Design review of the part built by this model. Coordinates are the model's own, in mm. A direction names the side the tool comes from. Coordinates: 2 decimals unless noted, no trailing zeros. Loops run counter-clockwise (first coordinate to the right, second up) from the corner with the lowest first, then second, coordinate; pieces in that order, holes last. Notation, with made-up numbers: (-39.75, 64.25) - (-2.75, 64.25) arc R20 ccw to (-2.75, 87.25) - close; hole circle Ø5 at (69.5, 29.25). An arc over 180 degrees is marked (long way). Use one line per item in the form item = value. Start each with the question number.
(1) Add section A-A (x = -1). State the section outline as (y, z) points, plus the area to 3 significant figures.
(2) For L1, parallel to X at y = 1.7, z = -4; L2, parallel to X at y = 3.75, z = -0.75; L3, parallel to Z at x = -0.5, y = 1.5, list the stretches that pass through material, from the lowest coordinate up.
(3) Tool access review of faces 1 (the face through (-4.5, 2, 0)), 2 (the face through (3.5, 2, 2)): name each direction out of +Z, -Z, +X, -X, +Y, -Y from which nothing blocks a thin tool from reaching the whole face with its end or side.
(4) Add section C-C (y = 0.6). State the section outline as (x, z) points.
(5) Add section D-D (z = -4). State the section outline as (x, y) points, plus the area to 3 significant figures.
(6) Add section B-B (x = 0). State the section outline as (y, z) points.
(7) Clearance check with a flat-ended pin moving along its axis: pin 1 Ø1 at (x, z) = (-0.5, -3.5) entering from -Y. State where the tip first meets the part, or that it passes through.
(8) The part is to be moulded in two halves that separate along Z. For faces 3 (the face through (0, 2, -2)), 4 (the face through (4.5, 2, 0)), 5 (the face through (4.199, 2.415, 5.715)), 6 (the face through (-3.215, 2.348, -1.699)), say which applies: pulls with the +Z half, pulls with the -Z half, needs draft (parallel to the pull), parting line crosses it, or undercut.
```python
from build123d import *

# Parameters (mm, degrees)
SKETCH1_W                           = 9
SKETCH1_H                           = 12
EXTRUDE1_DEPTH                      = 4.7625
SKETCH2_W                           = 7
SKETCH2_H                           = 7
EXTRUDE2_DEPTH                      = 5.7625
F_0_80_TAPPED_HOLE1_D               = 1.19126
F_3_32_0_09375_DIAMETER_HOLE1_D     = 2.38125
F_3_32_0_09375_DIAMETER_HOLE1_DEPTH = 10
F_3_32_0_09375_DIAMETER_HOLE1_TIP   = 0.715399675
FILLET7_R                           = 1


with BuildPart() as part:
    # Sketch1 → Extrude1 (new body)
    with BuildSketch(Plane(origin=(0, 0, 0), x_dir=(1, 0, 0), z_dir=(0, 1, 0))):
        Rectangle(SKETCH1_W, SKETCH1_H)
    extrude(amount=EXTRUDE1_DEPTH)

    # Sketch2 → Extrude2 (cut, through all)
    with BuildSketch(Plane(origin=(0, 4.7625, 0), x_dir=(1, 0, 0), z_dir=(0, 1, 0))):
        with Locations((0, -1.5)):
            Rectangle(SKETCH2_W, SKETCH2_H)
    extrude(amount=-EXTRUDE2_DEPTH, mode=Mode.SUBTRACT)

    # #0-80 Tapped Hole1 (through all)
    with Locations(Plane(origin=(0, 4.7625, -4), x_dir=(0, 0, 1), z_dir=(0, 1, 0))):
        with Locations((0, 0)):
            Hole(F_0_80_TAPPED_HOLE1_D / 2)

    # 3/32 (0.09375) Diameter Hole1
    with Locations(Plane(origin=(-2.5, 4.7625, -4), x_dir=(0, 0, 1), z_dir=(0, 1, 0))):
        with Locations((0, 0), (0, 5)):
            Hole(F_3_32_0_09375_DIAMETER_HOLE1_D / 2, depth=F_3_32_0_09375_DIAMETER_HOLE1_DEPTH)
            with Locations((0, 0, -(F_3_32_0_09375_DIAMETER_HOLE1_DEPTH + F_3_32_0_09375_DIAMETER_HOLE1_TIP / 2))):  # 118° drill point
                Cone(0, F_3_32_0_09375_DIAMETER_HOLE1_D / 2, F_3_32_0_09375_DIAMETER_HOLE1_TIP, mode=Mode.SUBTRACT)

    # Fillet7
    fillet7_edges = [part.edges().sort_by_distance(p)[0] for p in [
        (-3.5, 2.38125, 5),
        (-3.5, 2.38125, -2),
        (3.5, 2.38125, -2),
        (3.5, 2.38125, 5),
        (-4.5, 2.38125, -6),
        (4.5, 2.38125, -6),
        (4.5, 2.38125, 6),
        (-4.5, 2.38125, 6),
    ]]
    fillet(fillet7_edges, radius=FILLET7_R)


solid = part.part
```
Computed values:
q1.outline = (0, -6) - (4.76, -6) - (4.76, -2) - (0, -2) - close; (0, 5) - (4.76, 5) - (4.76, 6) - (0, 6) - close
q1.area = 23.8 mm^2
q2.L1 = -4.5 to -3.69, -1.31 to -0.6, 0.6 to 1.31, 3.69 to 4.5
q2.L2 = -4.5 to -3.5, 3.5 to 4.5
q2.L3 = -6 to -4.32, -3.68 to -2, 5 to 6
q3.face_1 = +Z, -Z, -X, +Y, -Y
q3.face_2 = +Y, -Y
q4.outline = (-4.5, -5) arc R1 ccw to (-3.5, -6) - (3.5, -6) arc R1 ccw to (4.5, -5) - (4.5, 5) arc R1 ccw to (3.5, 6) - (-3.5, 6) arc R1 ccw to (-4.5, 5) - close; hole circle Ø2.38 at (-2.5, -4); hole (-3.5, -1) arc R1 ccw to (-2.5, -2) - (2.5, -2) arc R1 ccw to (3.5, -1) - (3.5, 4) arc R1 ccw to (2.5, 5) - (-2.5, 5) arc R1 ccw to (-3.5, 4) - close; hole circle Ø1.19 at (0, -4); hole circle Ø2.38 at (2.5, -4)
q5.outline = (-4.5, 0) - (-3.69, 0) - (-3.69, 4.76) - (-4.5, 4.76) - close; (-1.31, 0) - (-0.6, 0) - (-0.6, 4.76) - (-1.31, 4.76) - close; (0.6, 0) - (1.31, 0) - (1.31, 4.76) - (0.6, 4.76) - close; (3.69, 0) - (4.5, 0) - (4.5, 4.76) - (3.69, 4.76) - close
q5.area = 14.5 mm^2
q6.outline = (0, -6) - (4.76, -6) - (4.76, -4.6) - (0, -4.6) - close; (0, -3.4) - (4.76, -3.4) - (4.76, -2) - (0, -2) - close; (0, 5) - (4.76, 5) - (4.76, 6) - (0, 6) - close
q7.pin_1 = 0
q8.face_3 = undercut
q8.face_4 = needs draft
q8.face_5 = pulls with the +Z half
q8.face_6 = undercut
